Read the model definition and answer for the solid it produces. Units are mm, in the model's axes. Face numbers are marked on the shaded views. A direction names the side the tool comes from. Coordinates: 2 decimals unless noted, no trailing zeros. Write each loop counter-clockwise with the first axis right and the second up, starting at its lowest first coordinate (ties: lowest second). Pieces come first, ordered by that corner, then holes.
Item 1: Section C-C (x = 16.5) is taken. Give the vertices of the cut face in (y, z).
Item 2: A tool of negligible diameter and unlimited length cuts with its end or side. For the marked faces 1, 2, 3 and 4, from which of +Z, -Z, +X, -X, +Y, -Y can it reach the whole face along a straight path? Write none if from no direction.
Item 3: Section B-B (z = 6.75) is taken. Give the vertices of the cut face in (x, y).
Item 4: Each of these flat-tipped pins is pushed along its axis until it touches: P1, Ø3, axis at y = -18, z = 5.5, coming from the +X side; P2, Ø0.9, axis at x = 25.5, z = 3, coming from the +Y side; P3, Ø2.5, axis at x = 20.5, z = 3, coming from the -Y side. Where does it stop, or does it pass through?
Item 5: Section A-A (x = 25) is taken. Give the vertices of the cut face in (y, z).
Item 6: Determine the mould class of the marked faces 5, 6 and 7 for opening direction Y: released by +Y, released by -Y, zero draft, split by the parting line, or undercut.
Item 7: Straight lines are drawn through the part: probe 1 along Y at (x, z) = (26, 1.5); probe 2 along X at (y, z) = (18, 7); probe 3 along Y at (x, z) = (15, 7). For each, find the intervals that lie inside material, in ascending order.
Item 8: Section D-D (y = 5) is taken. Give the vertices of the cut face in (x, z), then the cut area to 3 significant figures.
from build123d import *

# Parameters (mm, degrees)
BOSS_EXTRUDE1_DEPTH = 3
BOSS_EXTRUDE2_DEPTH = 5
SKETCH1_4_W         = 13
SKETCH1_4_H         = 10
BOSS_EXTRUDE3_DEPTH = 5
SKETCH2_W           = 3.1
SKETCH2_H           = 5.1
CUT_EXTRUDE1_DEPTH  = 6
BOSS_EXTRUDE4_DEPTH = 8
SKETCH3_W           = 13
SKETCH3_H           = 1.5
BOSS_EXTRUDE5_DEPTH = 2


with BuildPart() as part:
    # Sketch1 → Boss-Extrude1 (new body)
    with BuildSketch(Plane.XY):
        Polygon((9.93, 4.4), (13.6, 4.4), (13.6, 20.1), (-13.6, 20.1), (-13.6, 4.4), (-9.93, 4.4), (-9.93, -16.1), (-13.6, -16.1), (-13.6, -20.1), (-10, -20.1), (10, -20.1), (13.6, -20.1), (13.6, -16.1), (9.93, -16.1), align=None)
    extrude(amount=BOSS_EXTRUDE1_DEPTH)

    # Sketch1_3 → Boss-Extrude2 (add)
    with BuildSketch(Plane.XY):
        Polygon((15.6, 7.1), (15.6, 17.1), (15.6, 22.1), (-15.6, 22.1), (-15.6, 4.4), (-13.6, 4.4), (-13.6, 20.1), (13.6, 20.1), (13.6, 4.4), (15.6, 4.4), align=None)
        Polygon((15.6, -22.1), (15.6, -16.1), (13.6, -16.1), (13.6, -20.1), (10, -20.1), (10, -22.1), align=None)
        Polygon((-13.6, -16.1), (-15.6, -16.1), (-15.6, -22.1), (-10, -22.1), (-10, -20.1), (-13.6, -20.1), align=None)
    extrude(amount=BOSS_EXTRUDE2_DEPTH)

    # Sketch1_4 → Boss-Extrude3 (add)
    with BuildSketch(Plane.XY):
        with Locations((22.1, 12.1)):
            Rectangle(SKETCH1_4_W, SKETCH1_4_H)
    extrude(amount=BOSS_EXTRUDE3_DEPTH)

    # Sketch2 → Cut-Extrude1 (cut)
    with BuildSketch(Plane(origin=(28.6, 0, 0), x_dir=(0, 0, -1), z_dir=(1, 0, 0))):
        with Locations((-2.5, 12.1)):
            Rectangle(SKETCH2_W, SKETCH2_H)
    extrude(amount=-CUT_EXTRUDE1_DEPTH, mode=Mode.SUBTRACT)

    # Sketch1_5 → Boss-Extrude4 (add)
    with BuildSketch(Plane.XY):
        Polygon((15.6, 7.1), (15.6, 17.1), (15.6, 22.1), (-15.6, 22.1), (-15.6, 4.4), (-13.6, 4.4), (-13.6, 20.1), (13.6, 20.1), (13.6, 4.4), (15.6, 4.4), align=None)
        Polygon((-13.6, -16.1), (-15.6, -16.1), (-15.6, -22.1), (-10, -22.1), (-10, -20.1), (-13.6, -20.1), align=None)
        Polygon((15.6, -22.1), (15.6, -16.1), (13.6, -16.1), (13.6, -20.1), (10, -20.1), (10, -22.1), align=None)
    extrude(amount=BOSS_EXTRUDE4_DEPTH)

    # Sketch3 → Boss-Extrude5 (add)
    with BuildSketch(Plane(origin=(0, 0, 0), x_dir=(-1, 0, 0), z_dir=(0, 0, -1))):
        with Locations((-22.1, -16.85)):
            Rectangle(SKETCH3_W, SKETCH3_H)
    extrude(amount=-BOSS_EXTRUDE5_DEPTH)


solid = part.part
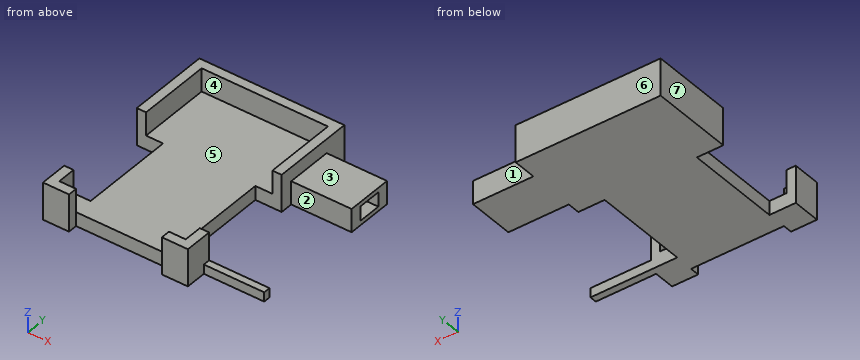
Established:
1. outline: (-17.6, 0) - (-16.1, 0) - (-16.1, 2) - (-17.6, 2) - close; (7.1, 0) - (17.1, 0) - (17.1, 5) - (7.1, 5) - close
2. face 1: +Z, -Z, +X, +Y
2. face 2: +Z, -Z, +X
2. face 3: +Z, +X, +Y, -Y
2. face 4: +Z
3. outline: (-15.6, -22.1) - (-10, -22.1) - (-10, -20.1) - (-13.6, -20.1) - (-13.6, -16.1) - (-15.6, -16.1) - close; (-15.6, 4.4) - (-13.6, 4.4) - (-13.6, 20.1) - (13.6, 20.1) - (13.6, 4.4) - (15.6, 4.4) - (15.6, 22.1) - (-15.6, 22.1) - close; (10, -22.1) - (15.6, -22.1) - (15.6, -16.1) - (13.6, -16.1) - (13.6, -20.1) - (10, -20.1) - close
4. P1: stops at x = 15.6
4. P2: stops at y = 17.1
4. P3: stops at y = -17.6
5. outline: (-17.6, 0) - (-16.1, 0) - (-16.1, 2) - (-17.6, 2) - close; (7.1, 0) - (17.1, 0) - (17.1, 5) - (7.1, 5) - close; hole (9.55, 0.95) - (14.65, 0.95) - (14.65, 4.05) - (9.55, 4.05) - close
6. face 5: undercut
6. face 6: released by +Y
6. face 7: zero draft
7. probe 1: y = -17.6 to -16.1, 7.1 to 9.55, 14.65 to 17.1
7. probe 2: x = -15.6 to -13.6, 13.6 to 15.6
7. probe 3: y = -22.1 to -16.1, 4.4 to 22.1
8. outline: (-15.6, 0) - (15.6, 0) - (15.6, 8) - (13.6, 8) - (13.6, 3) - (-13.6, 3) - (-13.6, 8) - (-15.6, 8) - close
8. area: 114 mm2
